The model under review builds one solid part; all positions refer to its coordinate system, in mm. A direction names the side the tool comes from. Round coordinates to 2 decimals unless told otherwise and drop trailing zeros. Loops run counter-clockwise (first coordinate to the right, second up) from the corner with the lowest first, then second, coordinate; pieces in that order, holes last. Notation, with made-up numbers: (-2, 3.25) -> (22, 3.25) arc R32 ccw to (22, 37.25) -> close; hole circle Ø7 at (-21, -2.5). An arc over 180 degrees is marked (long way). Use a Markdown table: item, result. Add a question column.
1) Consider section B-B on z = 0.25. Give the boundary of the cut face in (x, y), plus the area to 3 significant figures.
2) Consider section C-C on y = -3.75. Give the boundary of the cut face in (x, z).
3) Wall thickness on probe 1 along Z at (x, y) = (1, 4.25); probe 2 along X at (y, z) = (3.75, -2.75); probe 3 along Z at (x, y) = (-57, 4.25): over which ranges is each line inside the solid? List them lowest first.
4) Insertion check: pin 1 (5 mm diameter, centred on x = -19.5, y = 4, fed in from -Z); pin 2 (3 mm diameter, centred on x = -20.5, y = -0.5, fed in from +Z); pin 3 (2 mm diameter, centred on y = -3, z = 6.5, fed in from +X). Each pin has a flat end and moves straight along its axis. Give the tip position at first contact, or say it passes through.
5) Mouldability with a two-part tool opening along X and no side actions: class faces 1 (the flat face through (-71.023, 0, 0)), 2 (the flat face through (-32, 5, 0)), 3 (the flat face through (2, 0, -5)), 4 (the cylindrical face through (6.407, 0.451, 0.105)) as released by +X, released by -X, zero draft, split by the parting line, or undercut.
6) Consider section D-D on x = -51. Give the boundary of the cut face in (y, z).
7) For faces 5 (the flat face through (-1.023, 0, 7)), 6 (the flat face through (4.977, -3, 6)), 7 (the flat face through (4.977, 3, 6)), 8 (the flat face through (-36, 0, -6.25)), list the 3-axis set-ups (+Z, -Z, +X, -X, +Y, -Y) from which the entire face can be reached by the end or side of a thin tool; tool diameter is ignored.
8) Consider section A-A on y = 0. Give the boundary of the cut face in (x, z).
Autodesk Inventor part; units mm, degrees
ref_plane "YZ Plane" through (0, 0, 0) normal (1, 0, 0) x (0, 1, 0)
ref_plane "XZ Plane" through (0, 0, 0) normal (0, 1, 0) x (-1, 0, 0)
ref_plane "XY Plane" through (0, 0, 0) normal (0, 0, 1) x (1, 0, 0)
sketch "草圖1" plane through (0, 0, 0) normal (0, 1, 0) x (-1, 0, 0)
  line L0 (71.0233, 6.25) -> (1.0233, 6.25)
  line L1 (1.0233, 6.25) -> (1.0233, -6.25)
  line L2 (1.0233, -6.25) -> (71.0233, -6.25)
  line L3 (71.0233, -6.25) -> (71.0233, 6.25)
  line L4 (1.0233, 5) -> (-4.9767, 5)
  line L5 (-4.9767, 5) -> (-4.9767, 7.5)
  line L6 (-4.9767, 7.5) -> (1.0233, 7.5)
  line L7 (1.0233, 7.5) -> (1.0233, 5)
  line L8 (1.0233, -5) -> (-4.9767, -5)
  line L9 (-4.9767, -5) -> (-4.9767, -7.5)
  line L10 (-4.9767, -7.5) -> (1.0233, -7.5)
  line L11 (1.0233, -7.5) -> (1.0233, -5)
  point P0 (0, 0)
  point P1 (1.0233, 6.25)
  dimension "d0" = 6
  dimension "d2" = 5
  dimension "d3" = 10
  dimension "d4" = 2.5
  dimension "d5" = 12.5
  dimension "d6" = 6.25
  dimension "d7" = 70
extrude "擠出1" add sketch "草圖1" along normal mid plane 10
sketch "草圖2" plane through (-1.0233, 5, 7.5) normal (0, 0, 1) x (1, 0, 0)
  line L0 (6, -10) -> (6, 0)
  circle A0 centre (6, -5) radius 1.5
  point P0 (1.0233, -5)
  dimension "d10" = 3
extrude "擠出2" add sketch "草圖2" against normal up to surface (15 mm away)
properties part number "axis_rf"
Result set:
| question | item | result |
|---|---|---|
| 1 | outline | (-71.02, -5) -> (-1.02, -5) -> (-1.02, 5) -> (-71.02, 5) -> close; circle Ø3 at (4.98, 0) |
| 1 | area | 707 mm2 |
| 2 | outline | (-71.02, -6.25) -> (-1.02, -6.25) -> (-1.02, -7.5) -> (4.98, -7.5) -> (4.98, -5) -> (-1.02, -5) -> (-1.02, 5) -> (4.98, 5) -> (4.98, 7.5) -> (-1.02, 7.5) -> (-1.02, 6.25) -> (-71.02, 6.25) -> close |
| 3 | probe 1 | -7.5 to -5, 5 to 7.5 |
| 3 | probe 2 | -71.02 to -1.02 |
| 3 | probe 3 | -6.25 to 6.25 |
| 4 | pin 1 | z = -6.25 |
| 4 | pin 2 | z = 6.25 |
| 4 | pin 3 | x = 4.98 |
| 5 | face 1 | released by -X |
| 5 | face 2 | zero draft |
| 5 | face 3 | undercut |
| 5 | face 4 | undercut |
| 6 | outline | (-5, -6.25) -> (5, -6.25) -> (5, 6.25) -> (-5, 6.25) -> close |
| 7 | face 5 | +Z, -X, +Y, -Y |
| 7 | face 6 | +Z, -Z, +X, -Y |
| 7 | face 7 | +Z, -Z, +X, +Y |
| 7 | face 8 | -Z, -X, +Y, -Y |
| 8 | outline | (-71.02, -6.25) -> (-1.02, -6.25) -> (-1.02, -7.5) -> (6.48, -7.5) -> (6.48, 7.5) -> (-1.02, 7.5) -> (-1.02, 6.25) -> (-71.02, 6.25) -> close; hole (-1.02, -5) -> (3.48, -5) -> (3.48, 5) -> (-1.02, 5) -> close |
